The listing builds one solid part. Answer for the finished solid, in the listing's coordinates (mm). Face numbers are marked on the shaded views. A direction names the side the tool comes from. Give positions to 0.01 mm unless a question says otherwise; leave off trailing zeros. Write each loop counter-clockwise with the first axis right and the second up, starting at its lowest first coordinate (ties: lowest second). Pieces come first, ordered by that corner, then holes. Notation, with made-up numbers: (62.25, 51) - (79.25, 51) arc R23 cw to (79.25, 86) - close; hole circle Ø8 at (19.5, 17.5). An arc over 180 degrees is marked (long way). Use a Markdown table: item, result. Add a question column.
from build123d import *

# Parameters (mm, degrees)
RESSALTO_EXTRUS_O2_DEPTH = 25
ESBO_O3_W                = 7
ESBO_O3_H                = 20
CORTE_EXTRUS_O1_DEPTH    = 3
ESBO_O4_W                = 9.984895554
ESBO_O4_H                = 20
CORTE_EXTRUS_O2_DEPTH    = 4
ESBO_O5_R                = 1.5
CORTE_EXTRUS_O7_DEPTH    = 31.740852298
CORTE_EXTRUS_O8_DEPTH    = 3
CORTE_EXTRUS_O9_DEPTH    = 2
CORTE_EXTRUS_O11_DEPTH   = 3
RESSALTO_EXTRUS_O4_DEPTH = 7


with BuildPart() as part:
    # Esboço1 → Ressalto-extrusão2 (new body)
    with BuildSketch(Plane.XY):
        with BuildLine():
            Line((2.25, -0.4), (5.986651819, -0.4))
            Line((5.986651819, -0.4), (7.989993742, -0.4))
            ThreePointArc((7.989993742, -0.4), (-8, 0), (7.989993742, 0.4))
            Line((7.989993742, 0.4), (5.986651819, 0.4))
            Line((5.986651819, 0.4), (2.25, 0.4))
            Line((2.25, 0.4), (2.25, 1.299038106))
            Line((2.25, 1.299038106), (0, 2.598076211))
            Line((0, 2.598076211), (-2.25, 1.299038106))
            Line((-2.25, 1.299038106), (-2.25, -1.299038106))
            Line((-2.25, -1.299038106), (0, -2.598076211))
            Line((0, -2.598076211), (2.25, -1.299038106))
            Line((2.25, -1.299038106), (2.25, -0.4))
        make_face()
    extrude(amount=RESSALTO_EXTRUS_O2_DEPTH)

    # Esboço3 → Corte-extrusão1 (cut)
    with BuildSketch(Plane(origin=(0, 8, 0), x_dir=(1, 0, 0), z_dir=(0, 1, 0))):
        with Locations((4.489993742, -12.5)):
            Rectangle(ESBO_O3_W, ESBO_O3_H)
    extrude(amount=-CORTE_EXTRUS_O1_DEPTH, mode=Mode.SUBTRACT)

    # Esboço4 → Corte-extrusão2 (cut)
    with BuildSketch(Plane(origin=(0, -8, 0), x_dir=(1, 0, 0), z_dir=(0, 1, 0))):
        with Locations((5.982441519, -12.5)):
            Rectangle(ESBO_O4_W, ESBO_O4_H)
    extrude(amount=CORTE_EXTRUS_O2_DEPTH, mode=Mode.SUBTRACT)

    # Esboço5 → Corte-extrusão7 (cut, through all)
    with BuildSketch(Plane(origin=(0, -8, 0), x_dir=(1, 0, 0), z_dir=(0, 1, 0))):
        with Locations(Location((3.61749587, -6, 0), (0, 0, 155.736314367))):
            Circle(ESBO_O5_R)
        with Locations(Location((3.61749587, -19, 0), (0, 0, 155.736314367))):
            Circle(ESBO_O5_R)
    extrude(amount=CORTE_EXTRUS_O7_DEPTH, mode=Mode.SUBTRACT)

    # Esboço11 → Corte-extrusão8 (cut)
    with BuildSketch(Plane(origin=(0, 8, 0), x_dir=(1, 0, 0), z_dir=(0, 1, 0))):
        Polygon((0.989993742, -2.5), (0.489993742, -2.5), (0.489993742, -22.5), (0.989993742, -22.5), (12.059858903, -22.5), (12.059858903, -2.5), align=None)
    extrude(amount=-CORTE_EXTRUS_O8_DEPTH, mode=Mode.SUBTRACT)

    # Esboço12 → Corte-extrusão9 (cut)
    with BuildSketch(Plane(origin=(0, 5, 0), x_dir=(1, 0, 0), z_dir=(0, 1, 0))):
        Polygon((5.493884245, -9.25), (10.492692387, -9.25), (10.492692387, -2.75), (5.493884245, -2.75), (1.741107495, -2.75), (-0.135280879, -6), (1.741107495, -9.25), align=None)
        Polygon((5.493884245, -15.75), (1.741107495, -15.75), (-0.135280879, -19), (1.741107495, -22.25), (5.493884245, -22.25), (10.492692387, -22.25), (10.492692387, -15.75), align=None)
    extrude(amount=-CORTE_EXTRUS_O9_DEPTH, mode=Mode.SUBTRACT)

    # Esboço13 → Corte-extrusão11 (cut)
    with BuildSketch(Plane(origin=(0, 8, 0), x_dir=(1, 0, 0), z_dir=(0, 1, 0))):
        Polygon((0.489993742, -2.5), (-0.010006258, -2.5), (-0.010006258, -22.5), (0.489993742, -22.5), (15.48114744, -22.5), (15.48114744, -2.5), align=None)
    extrude(amount=-CORTE_EXTRUS_O11_DEPTH, mode=Mode.SUBTRACT)

    # Esboço14 → Ressalto-extrusão4 (add, symmetric)
    with BuildSketch(Plane.XY.offset(12.5)):
        Polygon((0, -2.598076211), (2.25, -1.299038106), (1.45, -1.299038106), (0, -2.136195996), (-1.85, -1.068097998), (-1.85, 1.068097998), (0, 2.136195996), (1.45, 1.299038106), (2.25, 1.299038106), (0, 2.598076211), (-2.25, 1.299038106), (-2.25, -1.299038106), align=None)
    extrude(amount=RESSALTO_EXTRUS_O4_DEPTH, both=True)


solid = part.part
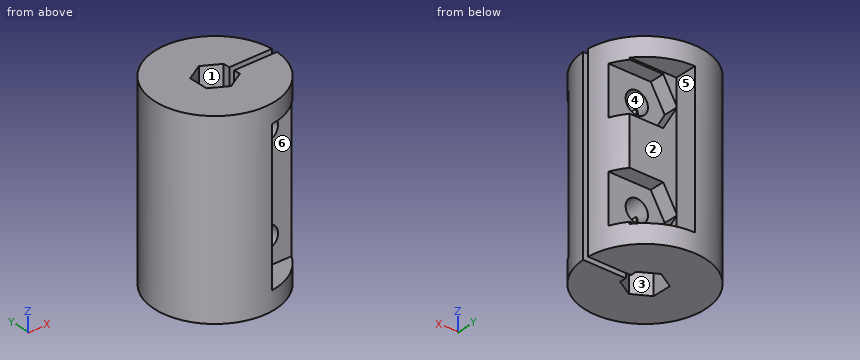
1. For a pull along X with two mould halves and no side action, classify the marked faces 4, 5 and 6 as released by +X, released by -X, zero draft, split by the parting line, or undercut.
2. Which of the six approach directions +Z, -Z, +X, -X, +Y, -Y give full straight-line access (tool end or side, diameter ignored) to the marked faces 1, 2 and 3?
3. Consider L1, parallel to Y at x = 5.25, z = 19.75; L2, parallel to X at y = 1.65, z = 6; L3, parallel to X at y = 1.55, z = 19. Determine where each line is inside the solid, lowest interval first. Write a range as [from, to].
4. The part is cut by section D-D (y = 0). Give the vertices of the cut face in (x, z).
5. Given P1, Ø1.5, axis at x = -1.5, z = 16, coming from the +Y side; P2, Ø1.8, axis at x = 3.62, z = 19, coming from the -Y side; P3, Ø3, axis at x = 4, y = -5, coming from the -Z side; P4, Ø1, axis at x = 5, z = 15.5, coming from the -Y side, each flat-ended and moving along its own axis, determine where each tip first touches the part or whether it passes through.
6. The part is cut by section A-A (y = 1.75). Give the vertices of the cut face in (x, z), and give its area (3 significant figures).
7. The part is cut by section C-C (y = -3.5). Give the vertices of the cut face in (x, z), and give its area (3 significant figures).
Check values:
| question | item | result |
|---|---|---|
| 1 | face 4 | undercut |
| 1 | face 5 | released by +X |
| 1 | face 6 | zero draft |
| 2 | face 1 | +Z |
| 2 | face 2 | +X, +Y |
| 2 | face 3 | -Z |
| 3 | L1 | y = [-4, -0.4], [0.4, 3] |
| 3 | L2 | x = [-7.83, -0.84], [0.84, 2.12], [5.12, 7.83] |
| 3 | L3 | x = [-7.85, -1.02], [1.02, 2.12], [5.12, 7.85] |
| 4 | outline | (-8, 0) - (-2.25, 0) - (-2.25, 5.5) - (-1.85, 5.5) - (-1.85, 19.5) - (-2.25, 19.5) - (-2.25, 25) - (-8, 25) - close |
| 5 | P1 | stops at y = 7.96 |
| 5 | P2 | passes through |
| 5 | P3 | stops at z = 0 |
| 5 | P4 | stops at y = -4 |
| 6 | outline | (-7.81, 0) - (-1.47, 0) - (-1.47, 5.5) - (-0.67, 5.5) - (-0.67, 19.5) - (-1.47, 19.5) - (-1.47, 25) - (-7.81, 25) - close; (0.67, 5.5) - (1.47, 5.5) - (1.47, 0) - (7.81, 0) - (7.81, 25) - (1.47, 25) - (1.47, 19.5) - (0.67, 19.5) - close; hole circle Ø3 at (3.62, 6); hole circle Ø3 at (3.62, 19) |
| 6 | area | 325 mm2 |
| 7 | outline | (-7.19, 0) - (7.19, 0) - (7.19, 25) - (-7.19, 25) - close; hole circle Ø3 at (3.62, 6); hole circle Ø3 at (3.62, 19) |
| 7 | area | 346 mm2 |
